from build123d import *

# Parameters (mm, degrees)
BOSS_EXTRUDE1_START                    = -9.525
SKETCH1_W                              = 170.984333333
SKETCH1_H                              = 247.65
BOSS_EXTRUDE1_DEPTH                    = 8.466666667
F_18_0_1695_DIAMETER_HOLE1_D           = 4.3053
F_18_0_1695_DIAMETER_HOLE1_CSINK_D     = 5.5753
F_18_0_1695_DIAMETER_HOLE1_CSINK_ANGLE = 90
BOTTOM_PINS_DEPTH                      = 6.35
REAR_PINS_DEPTH                        = 6.35
FRONT_PINS_DEPTH                       = 6.35
CUT_EXTRUDE1_DEPTH                     = 6.35
PIN_CHAMFERS_SIZE                      = 0.635


with BuildPart() as part:
    # Sketch1 → Boss-Extrude1 (new body)
    with BuildSketch(Plane.XY.offset(BOSS_EXTRUDE1_START)):
        with Locations((-38.078833334, 3.0734)):
            Rectangle(SKETCH1_W, SKETCH1_H)
        Polygon((-107.526666667, -116.518266667), (-107.526666667, -37.676666709), (-119.337666709, -25.865666667), (-119.337666709, 84.565066667), (38.946666667, 84.565066667), (38.946666667, -116.518266667), align=None, mode=Mode.SUBTRACT)
        Polygon((-119.337666709, 111.336666667), (-84.666666667, 111.336666667), (-77.5716, 118.431733333), (38.946666667, 118.431733333), (38.946666667, 88.7984), (-119.337666709, 88.7984), align=None, mode=Mode.SUBTRACT)
    extrude(amount=-BOSS_EXTRUDE1_DEPTH)

    # #18 (0.1695) Diameter Hole1 (through all)
    with Locations(Plane.XY.offset(-9.525)):
        with Locations((-88.9, 115.57), (43.18, 115.57), (43.18, -41.91), (43.18, -87.63), (43.18, -107.95), (-111.76, -87.63), (-111.76, -41.91)):
            CounterSinkHole(F_18_0_1695_DIAMETER_HOLE1_D / 2, F_18_0_1695_DIAMETER_HOLE1_CSINK_D / 2, counter_sink_angle=F_18_0_1695_DIAMETER_HOLE1_CSINK_ANGLE)

    # Sketch2 → bottom pins (cut)
    with BuildSketch(Plane.XZ.offset(120.7516)):
        Polygon((-122.512666667, -13.758333333), (-119.337666667, -10.583333333), (-116.162666667, -13.758333333), (-119.337666667, -16.933333333), align=None)
        Polygon((40.005, -13.758333333), (43.18, -10.583333333), (46.355, -13.758333333), (43.18, -16.933333333), align=None)
    extrude(amount=-BOTTOM_PINS_DEPTH, mode=Mode.SUBTRACT)

    # Sketch3 → rear pins (cut)
    with BuildSketch(Plane.ZY.offset(123.571)):
        Polygon((-16.933333333, 115.57), (-13.758333333, 118.745), (-10.583333333, 115.57), (-13.758333333, 112.395), align=None)
    extrude(amount=-REAR_PINS_DEPTH, mode=Mode.SUBTRACT)

    # Sketch4 → front pins (cut)
    with BuildSketch(Plane(origin=(47.413333333, 0, 0), x_dir=(0, 0, -1), z_dir=(1, 0, 0))):
        Polygon((10.583333333, 122.665066667), (13.758333333, 125.840066667), (16.933333333, 122.665066667), (13.758333333, 119.490066667), align=None)
        Polygon((10.583333333, -97.8916), (13.758333333, -94.7166), (16.933333333, -97.8916), (13.758333333, -101.0666), align=None)
    extrude(amount=-FRONT_PINS_DEPTH, mode=Mode.SUBTRACT)

    # Sketch7 → Cut-Extrude1 (cut)
    with BuildSketch(Plane(origin=(0, 126.8984, 0), x_dir=(1, 0, 0), z_dir=(0, 1, 0))):
        Polygon((-6.095999915, 13.758333333), (-9.270999915, 10.583333333), (-12.445999915, 13.758333333), (-9.270999915, 16.933333333), align=None)
        Polygon((-116.162666667, 13.758333333), (-119.337666667, 10.583333333), (-122.512666667, 13.758333333), (-119.337666667, 16.933333333), align=None)
        Polygon((0.254000085, 13.758333333), (3.429000085, 16.933333333), (6.604000085, 13.758333333), (3.429000085, 10.583333333), align=None)
    extrude(amount=-CUT_EXTRUDE1_DEPTH, mode=Mode.SUBTRACT)

    # pin chamfers
    pin_chamfers_edges = [part.edges().sort_by_distance(p)[0] for p in [
        (-120.925166667, -114.4016, -15.345833333),
        (-120.925166667, -114.4016, -12.170833333),
        (-117.750166667, -114.4016, -12.170833333),
        (-117.750166667, -114.4016, -15.345833333),
        (-120.925166667, -120.7516, -15.345833333),
        (-117.750166667, -120.7516, -15.345833333),
        (-117.750166667, -120.7516, -12.170833333),
        (-120.925166667, -120.7516, -12.170833333),
        (41.5925, -114.4016, -15.345833333),
        (41.5925, -114.4016, -12.170833333),
        (44.7675, -114.4016, -12.170833333),
        (44.7675, -114.4016, -15.345833333),
        (41.5925, -120.7516, -15.345833333),
        (44.7675, -120.7516, -15.345833333),
        (44.7675, -120.7516, -12.170833333),
        (41.5925, -120.7516, -12.170833333),
        (-117.221, 113.9825, -15.345833333),
        (-117.221, 117.1575, -15.345833333),
        (-117.221, 117.1575, -12.170833333),
        (-117.221, 113.9825, -12.170833333),
        (-123.571, 113.9825, -15.345833333),
        (-123.571, 113.9825, -12.170833333),
        (-123.571, 117.1575, -12.170833333),
        (-123.571, 117.1575, -15.345833333),
        (41.063333333, 121.077566667, -12.170833333),
        (41.063333333, 124.252566667, -12.170833333),
        (41.063333333, 124.252566667, -15.345833333),
        (41.063333333, 121.077566667, -15.345833333),
        (47.413333333, 121.077566667, -12.170833333),
        (47.413333333, 121.077566667, -15.345833333),
        (47.413333333, 124.252566667, -15.345833333),
        (47.413333333, 124.252566667, -12.170833333),
        (41.063333333, -99.4791, -12.170833333),
        (41.063333333, -96.3041, -12.170833333),
        (41.063333333, -96.3041, -15.345833333),
        (41.063333333, -99.4791, -15.345833333),
        (47.413333333, -99.4791, -12.170833333),
        (47.413333333, -99.4791, -15.345833333),
        (47.413333333, -96.3041, -15.345833333),
        (47.413333333, -96.3041, -12.170833333),
        (1.841500085, 120.5484, -12.170833333),
        (1.841500085, 120.5484, -15.345833333),
        (5.016500085, 120.5484, -15.345833333),
        (5.016500085, 120.5484, -12.170833333),
        (1.841500085, 126.8984, -12.170833333),
        (5.016500085, 126.8984, -12.170833333),
        (5.016500085, 126.8984, -15.345833333),
        (1.841500085, 126.8984, -15.345833333),
        (-117.750166667, 120.5484, -15.345833333),
        (-117.750166667, 120.5484, -12.170833333),
        (-120.925166667, 120.5484, -12.170833333),
        (-120.925166667, 120.5484, -15.345833333),
        (-117.750166667, 126.8984, -15.345833333),
        (-120.925166667, 126.8984, -15.345833333),
        (-120.925166667, 126.8984, -12.170833333),
        (-117.750166667, 126.8984, -12.170833333),
        (-7.683499915, 120.5484, -15.345833333),
        (-7.683499915, 120.5484, -12.170833333),
        (-10.858499915, 120.5484, -12.170833333),
        (-10.858499915, 120.5484, -15.345833333),
        (-7.683499915, 126.8984, -15.345833333),
        (-10.858499915, 126.8984, -15.345833333),
        (-10.858499915, 126.8984, -12.170833333),
        (-7.683499915, 126.8984, -12.170833333),
    ]]
    chamfer(pin_chamfers_edges, length=PIN_CHAMFERS_SIZE)


solid = part.part
Input: part model. Units: mm. Frame: model coordinates. A direction names the side the tool comes from. Give positions to 0.01 mm unless a question says otherwise; leave off trailing zeros. Order: outer loops, then holes, each group sorted by start corner. A loop starts at its lowest first (then second) coordinate and runs counter-clockwise, first axis right, second up. Notation, with made-up numbers: (25, 39.5) - (53, 39.5) arc R9 ccw to (53, 52.5) - close; hole circle Ø6 at (34, 47). An arc over 180 degrees is marked (long way). Answer as a JSON object with one key per item and string values. Group by question number.
Q1. Mould query, pull axis X, two halves, no side actions, for faces 4 (the face through (-39, -120.752, -14)), 5 (the face through (47.413, 1, -14)), 6 (the face through (-107.527, -78, -14)). Classes: pulls with the +X half, pulls with the -X half, needs draft (parallel to the pull), parting line crosses it, or undercut.
Q2. Cut plane A-A, the plane y = 43. Output: boundary loops of the cut face in (x, z) (3 decimals).
Q3. Line query: probe 1 along Y at (x, z) = (-66, -11.25); probe 2 along X at (y, z) = (-107.95, -12.5); probe 3 along Y at (x, z) = (-94, -9.75). Output: solid intervals per line, ascending.
Q4. Set-up query: faces 1 (the face through (-33, -116.518, -14)), 2 (the face through (-119, 120.548, -14)), 3 (the face through (-119, -114.402, -14)). Return all of +Z, -Z, +X, -X, +Y, -Y with unobstructed straight access to the full face (end or side cutting, diameter ignored); none if empty.
Q5. First-contact query: pin 1 Ø1.5 at (x, y) = (-33, 82.5) entering from +Z; pin 2 Ø1.4 at (x, z) = (3, -13) entering from +Y; pin 3 Ø3.5 at (x, z) = (43.5, -14.5) entering from -Y; pin 4 Ø2.5 at (x, z) = (-10, -13.5) entering from +Y. Flat tips, straight axial feed; report the tip coordinate or a pass-through.
Q6. Cut plane B-B, the plane x = -70. Output: boundary loops of the cut face in (y, z) (3 decimals), then the cut area to 3 significant figures.
Results:
{
 "1": {"face 4": "needs draft", "face 5": "pulls with the +X half", "face 6": "undercut"},
 "2": {"outline": "(-123.571, -17.992) - (-119.338, -17.992) - (-119.338, -9.525) - (-123.571, -9.525) - close; (38.947, -17.992) - (47.413, -17.992) - (47.413, -9.525) - (38.947, -9.525) - close"},
 "3": {"probe 1": "-120.75 to -116.52, 84.57 to 88.8, 118.43 to 126.9", "probe 2": "-123.57 to -107.53, 38.95 to 41.03, 45.33 to 47.41", "probe 3": "-120.75 to -116.52, 84.57 to 88.8, 111.34 to 126.9"},
 "4": {"face 1": "+Z, -Z", "face 2": "+Y", "face 3": "-Y"},
 "5": {"pin 1": "through", "pin 2": "y = 120.55", "pin 3": "y = -120.37", "pin 4": "y = 120.89"},
 "6": {"outline": "(-120.752, -17.992) - (-116.518, -17.992) - (-116.518, -9.525) - (-120.752, -9.525) - close; (84.565, -17.992) - (88.798, -17.992) - (88.798, -9.525) - (84.565, -9.525) - close; (118.432, -17.992) - (126.898, -17.992) - (126.898, -9.525) - (118.432, -9.525) - close", "area": "143 mm^2"}
}
